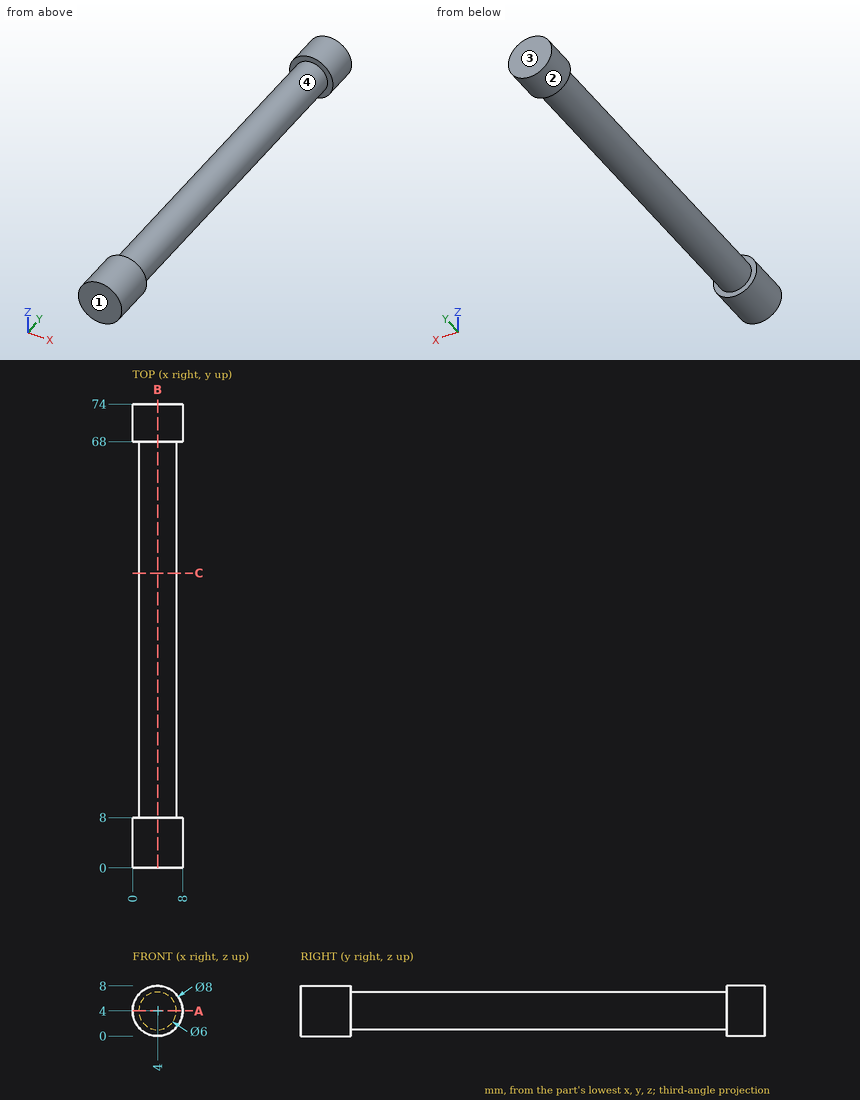
Drawing for the job (mm, zero at the part's lowest x, y, z). Give positions to 0.01 mm unless a question says otherwise; leave off trailing zeros. Order: outer loops, then holes, each group sorted by start corner. A loop starts at its lowest first (then second) coordinate and runs counter-clockwise, first axis right, second up. Notation, with made-up numbers: (12.25, -29.75) -> (18.25, -29.75) arc R16 ccw to (18.25, -14.75) -> close; hole circle Ø9 at (-16, -8). An arc over 180 degrees is marked (long way). Use one line per item in the form item = value.
(1) Flat gauge pins, fed straight in: P1, Ø2, axis at y = 57.5, z = 4, coming from the +X side; P2, Ø2, axis at y = 27, z = 5, coming from the -X side; P3, Ø3, axis at x = 1.5, y = 42, coming from the -Z side. Where does each tip first touch, or does it go through?
Solution:
P1 = 7
P2 = 1
P3 = 1.17
(2) Saw through at B-B (x = 4). Write the cut outline in (y, z), then the cut area to 3 significant figures.
Solution:
outline = (0, 0) -> (8, 0) -> (8, 1) -> (68, 1) -> (68, 0) -> (74, 0) -> (74, 8) -> (68, 8) -> (68, 7) -> (8, 7) -> (8, 8) -> (0, 8) -> close
area = 472 mm²
(3) Saw through at C-C (y = 47). Write the cut outline in (x, z), then the cut area to 3 significant figures.
Solution:
outline = circle Ø6 at (4, 4)
area = 28.3 mm²
(4) Pull direction Y, two halves, no side cores. Call the marked faces 1, 2, 3 and 4: +Y half, -Y half, draft (parallel to the pull), parting line (faces both ways), or undercut.
Solution:
face_1 = -Y half
face_2 = draft
face_3 = +Y half
face_4 = undercut
(5) Drill centre lines: line 1 (Y direction, x = 7.5, z = 2.75); line 2 (Z direction, x = 1.25, y = 70.5); line 3 (X direction, y = 50.5, z = 3.75). Where is each one in solid material? Low to high. Write a range as from..to.
Solution:
line_1 = 0..8, 68..74
line_2 = 1.1..6.9
line_3 = 1.01..6.99
(6) Saw through at A-A (z = 4). Write the cut outline in (x, y).
Solution:
outline = (0, 0) -> (8, 0) -> (8, 8) -> (7, 8) -> (7, 68) -> (8, 68) -> (8, 74) -> (0, 74) -> (0, 68) -> (1, 68) -> (1, 8) -> (0, 8) -> close
